```python
from build123d import *

# Parameters (mm, degrees)
ESQUISSE1_W                             = 33
ESQUISSE1_H                             = 39
BOSS_EXTRU_1_DEPTH                      = 1.5
ESQUISSE2_W                             = 39
ESQUISSE2_H                             = 33
ESQUISSE2_W_2                           = 36
ESQUISSE2_H_2                           = 30
BOSS_EXTRU_2_DEPTH                      = 19
ESQUISSE3_W                             = 27
ESQUISSE3_H                             = 4.6
BOSS_EXTRU_3_DEPTH                      = 11
ESQUISSE5_W                             = 26
ESQUISSE5_H                             = 0.65
BOSS_EXTRU_4_DEPTH                      = 3.4
ESQUISSE10_W                            = 0.5
ESQUISSE10_H                            = 20.8
ESQUISSE10_W_2                          = 1
ESQUISSE10_H_2                          = 3
BOSS_EXTRU_5_DEPTH                      = 5
ESQUISSE12_W                            = 10.05
ESQUISSE12_H                            = 3.4
ENL_V_MAT_EXTRU_5_DEPTH                 = 46.403744339
ESQUISSE13_W                            = 7
ESQUISSE13_H                            = 13.8
BOSS_EXTRU_6_DEPTH                      = 5.4
ESQUISSE14_W                            = 6
ESQUISSE14_H                            = 11.8
ENL_V_MAT_EXTRU_6_DEPTH                 = 2
ESQUISSE15_W                            = 5
ESQUISSE15_H                            = 2.3
ENL_V_MAT_EXTRU_7_DEPTH                 = 46.812116301
ENL_VEMENT_DE_MATI_RE_R_VOLUTION5_ANGLE = 180
SYM_TRIE4_COPY_1_ANGLE                  = 180
ESQUISSE17_W                            = 10
ESQUISSE17_H                            = 1
ENL_V_MAT_EXTRU_8_DEPTH                 = 48.047847985
CONG_1_R                                = 1
ESQUISSE18_W                            = 7.595753743
ESQUISSE18_H                            = 2.860925691
ENL_V_MAT_EXTRU_9_DEPTH                 = 32.835514759
ESQUISSE19_W                            = 2.860925691
ESQUISSE19_H                            = 3
ENL_V_MAT_EXTRU_10_DEPTH                = 46.403744339


with BuildPart() as part:
    # Esquisse1 → Boss.-Extru.1 (new body)
    with BuildSketch(Plane(origin=(0, 0, 0), x_dir=(0, 1, 0), z_dir=(0, 0, 1))):
        Rectangle(ESQUISSE1_W, ESQUISSE1_H)
    extrude(amount=BOSS_EXTRU_1_DEPTH)

    # Esquisse2 → Boss.-Extru.2 (add)
    with BuildSketch(Plane.XY.offset(1.5)):
        Rectangle(ESQUISSE2_W, ESQUISSE2_H)
        Rectangle(ESQUISSE2_W_2, ESQUISSE2_H_2, mode=Mode.SUBTRACT)
    extrude(amount=BOSS_EXTRU_2_DEPTH)

    # Esquisse3 → Boss.-Extru.3 (add)
    with BuildSketch(Plane.XY.offset(1.5)):
        with Locations((-4.5, 12.7)):
            Rectangle(ESQUISSE3_W, ESQUISSE3_H)
        with Locations((-4.5, -12.7)):
            Rectangle(ESQUISSE3_W, ESQUISSE3_H)
    extrude(amount=BOSS_EXTRU_3_DEPTH)

    # Esquisse5 → Boss.-Extru.4 (add)
    with BuildSketch(Plane.XY.offset(1.5)):
        with Locations((-5, 10.075)):
            Rectangle(ESQUISSE5_W, ESQUISSE5_H)
        with Locations((-5, -10.075)):
            Rectangle(ESQUISSE5_W, ESQUISSE5_H)
    extrude(amount=BOSS_EXTRU_4_DEPTH)

    # Esquisse10 → Boss.-Extru.5 (add)
    with BuildSketch(Plane.XY.offset(1.5)):
        with Locations((-17.75, 0)):
            Rectangle(ESQUISSE10_W, ESQUISSE10_H)
        with Locations((8.5, 8.9)):
            Rectangle(ESQUISSE10_W_2, ESQUISSE10_H_2)
        with Locations((8.5, -8.9)):
            Rectangle(ESQUISSE10_W_2, ESQUISSE10_H_2)
    extrude(amount=BOSS_EXTRU_5_DEPTH)

    # Esquisse12 → Enlèv. mat.-Extru.5 (cut, through all)
    with BuildSketch(Plane.YZ.offset(-17.5)):
        with Locations((0, 3.2)):
            Rectangle(ESQUISSE12_W, ESQUISSE12_H)
    extrude(amount=-ENL_V_MAT_EXTRU_5_DEPTH, mode=Mode.SUBTRACT)

    # Esquisse13 → Boss.-Extru.6 (add)
    with BuildSketch(Plane(origin=(-15.623853211, 9.112155963, 1.5), x_dir=(1, 0, 0), z_dir=(0, 0, 1))):
        with Locations((30.123853211, -9.112155963)):
            Rectangle(ESQUISSE13_W, ESQUISSE13_H)
    extrude(amount=BOSS_EXTRU_6_DEPTH)

    # Esquisse14 → Enlèv. mat.-Extru.6 (cut)
    with BuildSketch(Plane.XY.offset(6.9)):
        with Locations((15, 0)):
            Rectangle(ESQUISSE14_W, ESQUISSE14_H)
    extrude(amount=-ENL_V_MAT_EXTRU_6_DEPTH, mode=Mode.SUBTRACT)

    # Esquisse15 → Enlèv. mat.-Extru.7 (cut, through all)
    with BuildSketch(Plane(origin=(18, 0, 0), x_dir=(0, -1, 0), z_dir=(-1, 0, 0))):
        with Locations((0, 6.65)):
            Rectangle(ESQUISSE15_W, ESQUISSE15_H)
    extrude(amount=-ENL_V_MAT_EXTRU_7_DEPTH, mode=Mode.SUBTRACT)

    # Esquisse16 → Enlèvement de matière-Révolution5 (revolve, cut)
    with BuildSketch(Plane.XZ.offset(-14.96)):
        with BuildLine():
            Line((-8.65, 20), (-9.35, 20))
            ThreePointArc((-9.35, 20), (-9, 20.35), (-8.65, 20))
        make_face()
    enl_vement_de_mati_re_r_volution5 = revolve(axis=Axis((-14.897028004, 14.96, 20), (-1, 0, 0)), revolution_arc=ENL_VEMENT_DE_MATI_RE_R_VOLUTION5_ANGLE, mode=Mode.SUBTRACT)

    # Symétrie3: Enlèvement de matière-Révolution5 across plane
    add(enl_vement_de_mati_re_r_volution5.mirror(Plane.ZX), mode=Mode.SUBTRACT)

    # Symétrie4: Enlèvement de matière-Révolution5 across plane
    add(enl_vement_de_mati_re_r_volution5.mirror(Plane(origin=(0, 0, 0), x_dir=(0, 0, 1), z_dir=(1, 0, 0))), mode=Mode.SUBTRACT)

    # Symétrie4 copy 1 sketch → Symétrie4 copy 1 (revolve, cut)
    with BuildSketch(Plane(origin=(0, -14.96, 0), x_dir=(-1, 0, 0), z_dir=(0, 1, 0))):
        with BuildLine():
            Line((-8.65, 20), (-9.35, 20))
            ThreePointArc((-9.35, 20), (-9, 20.35), (-8.65, 20))
        make_face()
    revolve(axis=Axis((14.897028004, -14.96, 20), (1, 0, 0)), revolution_arc=SYM_TRIE4_COPY_1_ANGLE, mode=Mode.SUBTRACT)

    # Esquisse17 → Enlèv. mat.-Extru.8 (cut, through all)
    with BuildSketch(Plane(origin=(-19.5, 0, 0), x_dir=(0, -1, 0), z_dir=(-1, 0, 0))):
        with Locations((2.694173084, 20)):
            Rectangle(ESQUISSE17_W, ESQUISSE17_H)
    extrude(amount=-ENL_V_MAT_EXTRU_8_DEPTH, mode=Mode.SUBTRACT)

    # Congé1
    cong_1_edges = [part.edges().sort_by_distance(p)[0] for p in [
        (-19.5, -16.5, 10.25),
        (-19.5, 16.5, 10.25),
        (19.5, 16.5, 10.25),
        (19.5, -16.5, 10.25),
    ]]
    fillet(cong_1_edges, radius=CONG_1_R)

    # Esquisse18 → Enlèv. mat.-Extru.9 (cut, through all)
    with BuildSketch(Plane.XY.offset(1.5)):
        with Locations((-13.702123129, 7.455462846)):
            Rectangle(ESQUISSE18_W, ESQUISSE18_H)
        with Locations((-13.702123129, -7.455462846)):
            Rectangle(ESQUISSE18_W, ESQUISSE18_H)
    extrude(amount=-ENL_V_MAT_EXTRU_9_DEPTH, mode=Mode.SUBTRACT)

    # Esquisse19 → Enlèv. mat.-Extru.10 (cut, through all)
    with BuildSketch(Plane.YZ.offset(-17.5)):
        with Locations((-7.455462846, 1.5)):
            Rectangle(ESQUISSE19_W, ESQUISSE19_H)
        with Locations((7.455462846, 1.5)):
            Rectangle(ESQUISSE19_W, ESQUISSE19_H)
    extrude(amount=-ENL_V_MAT_EXTRU_10_DEPTH, mode=Mode.SUBTRACT)


solid = part.part
```
Geometry check sheet. Reference: the model listing, model coordinates, mm. A direction names the side the tool comes from. Coordinates: 2 decimals unless noted, no trailing zeros. Loops run counter-clockwise (first coordinate to the right, second up) from the corner with the lowest first, then second, coordinate; pieces in that order, holes last. Notation, with made-up numbers: (-34.75, 87) -> (24.25, 87) arc R22 cw to (24.25, 125) -> close; hole circle Ø6 at (67.5, -2). An arc over 180 degrees is marked (long way). Put each result on its own line as item: value.
1) Gauge pin test, flat ends, axial feed: pin 1 Ø1.2 at (y, z) = (7.5, 1) entering from -X; pin 2 Ø2 at (x, y) = (-2.5, 0) entering from +Z; pin 3 Ø2 at (x, y) = (13.5, -2) entering from +Z. Record the tip position at first contact, or that the pin passes through.
Result set:
pin 1: stops at x = -9.9
pin 2: stops at z = 1.5
pin 3: stops at z = 4.9
2) Release check for a two-part mould opening along X. For faces 6 (the flat face through (12, 0, 6)), 7 (the flat face through (8.5, -8.9, 6.5)), 8 (the cylindrical face through (-19.215, -16.199, 10.394)), 9 (the flat face through (-19, -7.694, 20)) record: released by +X, released by -X, zero draft, split by the parting line, or undercut.
Result set:
face 6: undercut
face 7: undercut
face 8: released by -X
face 9: zero draft
3) Cross-section at C-C on y = 4. Record the boundary of the cut face in (x, z), plus the area to 3 significant figures.
Result set:
outline: (-19.5, 0) -> (19.5, 0) -> (19.5, 20.5) -> (18, 20.5) -> (18, 4.9) -> (12, 4.9) -> (12, 6.9) -> (11, 6.9) -> (11, 1.5) -> (-19.5, 1.5) -> close; (-19.5, 4.9) -> (-17.5, 4.9) -> (-17.5, 6.5) -> (-18, 6.5) -> (-18, 20.5) -> (-19.5, 20.5) -> close
area: 137 mm^2
4) Thickness scan on line 1 (X direction, y = 4, z = 5); line 2 (Y direction, x = 16, z = 9.5); line 3 (X direction, y = 12.5, z = 7.5). Record the ranges inside material, lowest first.
Result set:
line 1: x = -19.5 to -17.5, 11 to 12, 18 to 19.5
line 2: y = -16.5 to -15, 15 to 16.5
line 3: x = -19.5 to 9, 18 to 19.5
5) Tool access check on faces 1 (the flat face through (-19, 2.306, 20)), 2 (the flat face through (-16, -6.025, 1)), 3 (the flat face through (-18, -5.025, 3)), 4 (the flat face through (11.6, 0, 6.9)), 5 (the flat face through (19, 0, 5.5)). Record the directions out of +Z, -Z, +X, -X, +Y, -Y that give a thin tool (end or side, any length) a straight path to the whole face; none if there is none.
Result set:
face 1: +Z, +X, -X
face 2: -Z, -X
face 3: -X
face 4: +Z
face 5: +X
6) Cross-section at B-B on z = 9.25. Record the boundary of the cut face in (x, y), plus the area to 3 significant figures.
Result set:
outline: (-19.5, -15.5) arc R1 ccw to (-18.5, -16.5) -> (18.5, -16.5) arc R1 ccw to (19.5, -15.5) -> (19.5, 15.5) arc R1 ccw to (18.5, 16.5) -> (-18.5, 16.5) arc R1 ccw to (-19.5, 15.5) -> close; hole (-18, -10.4) -> (9, -10.4) -> (9, -15) -> (18, -15) -> (18, 15) -> (9, 15) -> (9, 10.4) -> (-18, 10.4) -> close
area: 455 mm^2
7) Cross-section at D-D on x = 13. Record the boundary of the cut face in (y, z).
Result set:
outline: (-16.5, 0) -> (16.5, 0) -> (16.5, 20.5) -> (15, 20.5) -> (15, 1.5) -> (6.9, 1.5) -> (6.9, 6.9) -> (5.9, 6.9) -> (5.9, 4.9) -> (-5.9, 4.9) -> (-5.9, 6.9) -> (-6.9, 6.9) -> (-6.9, 1.5) -> (-15, 1.5) -> (-15, 20.5) -> (-16.5, 20.5) -> close
8) Cross-section at A-A on y = -0.5. Record the boundary of the cut face in (x, z), plus the area to 3 significant figures.
Result set:
outline: (-19.5, 0) -> (19.5, 0) -> (19.5, 5.5) -> (18, 5.5) -> (18, 4.9) -> (12, 4.9) -> (12, 6.9) -> (11, 6.9) -> (11, 1.5) -> (-19.5, 1.5) -> close; (-19.5, 4.9) -> (-17.5, 4.9) -> (-17.5, 6.5) -> (-18, 6.5) -> (-18, 19.5) -> (-19.5, 19.5) -> close; (18, 7.8) -> (19.5, 7.8) -> (19.5, 19.5) -> (18, 19.5) -> close
area: 131 mm^2
